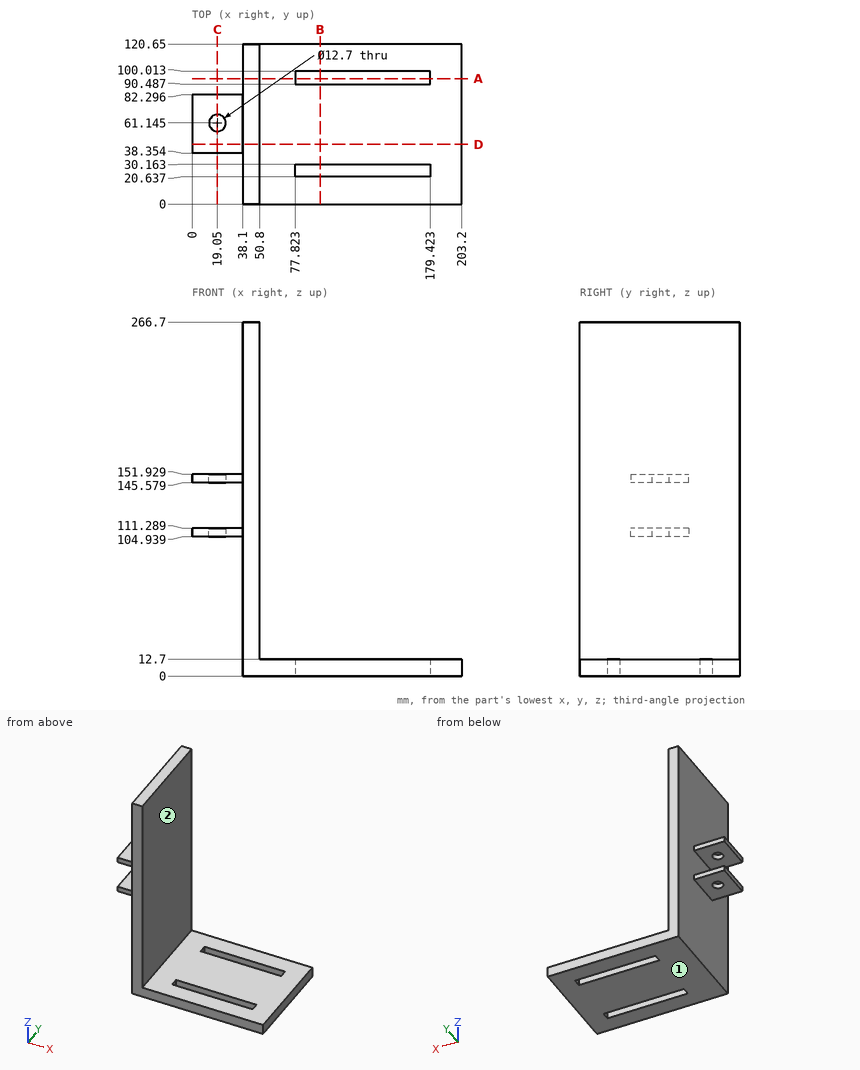
Could you check a few things on this drawing? It's one solid part, dimensions in mm from its lowest x, y, z. A direction names the side the tool comes from. Give positions to 0.01 mm unless a question says otherwise; leave off trailing zeros. Write each loop counter-clockwise with the first axis right and the second up, starting at its lowest first coordinate (ties: lowest second). Pieces come first, ordered by that corner, then holes. Notation, with made-up numbers: M 17.25,73 L 30.25,73 A24 cw 30.25,111 Z; hole C -18,-33 d4. An arc over 180 degrees is marked long. Put each result on its own line as item: value. Start each with the question number.
Item 1: If we section it at A-A, the plane y = 94.5: Write out the boundary of the cut face in (x, z), then the cut area to 3 significant figures.
Item 2: Will these pins go through, and if not, where does the flat tip stop? pin 1 (20.5 mm diameter, centred on x = 19.05, y = 61.15, fed in from +Z); pin 2 (19 mm diameter, centred on x = 26.5, y = 55, fed in from -Z); pin 3 (7 mm diameter, centred on x = 22, z = 108.5, fed in from -Y).
Item 3: If we section it at B-B, the plane x = 96.5: Write out the boundary of the cut face in (y, z), then the cut area to 3 significant figures.
Item 4: On a 3-axis mill with a long thin cutter (end or side, diameter ignored), from which of +Z, -Z, +X, -X, +Y, -Y can I reach the whole of each face in a straight line? I mean the marked faces 1 and 2. Say none if no direction works.
Item 5: I need wall thicknesses on L1, parallel to Y at x = 19.05, z = 149.25 (1 decimal); L2, parallel to X at y = 79, z = 162.5; L3, parallel to Z at x = 143, y = 30.5. Which ranges of each line are inside material? Lowest first, please. Write a range as from..to.
Item 6: If we section it at D-D, the plane y = 45: Write out the boundary of the cut face in (x, z), then the cut area to 3 significant figures.
Item 7: If we section it at C-C, the plane x = 19.05: Write out the boundary of the cut face in (y, z) (1 decimal).
Values:
1. outline: M 38.1,0 L 77.82,0 L 77.82,12.7 L 50.8,12.7 L 50.8,266.7 L 38.1,266.7 Z; M 179.42,0 L 203.2,0 L 203.2,12.7 L 179.42,12.7 Z
1. area: 4,030 mm²
2. pin 1: z = 151.93
2. pin 2: z = 104.94
2. pin 3: y = 38.35
3. outline: M 0,0 L 20.64,0 L 20.64,12.7 L 0,12.7 Z; M 30.16,0 L 90.49,0 L 90.49,12.7 L 30.16,12.7 Z; M 100.01,0 L 120.65,0 L 120.65,12.7 L 100.01,12.7 Z
3. area: 1,290 mm²
4. face 1: -Z, +X, -X, +Y, -Y
4. face 2: +Z, +X, +Y, -Y
5. L1: 38.4..54.8, 67.5..82.3
5. L2: 38.1..50.8
5. L3: 0..12.7
6. outline: M 0,104.94 L 38.1,104.94 L 38.1,0 L 203.2,0 L 203.2,12.7 L 50.8,12.7 L 50.8,266.7 L 38.1,266.7 L 38.1,151.93 L 0,151.93 L 0,145.58 L 38.1,145.58 L 38.1,111.29 L 0,111.29 Z
6. area: 5,810 mm²
7. outline: M 38.4,104.9 L 54.8,104.9 L 54.8,111.3 L 38.4,111.3 Z; M 38.4,145.6 L 54.8,145.6 L 54.8,151.9 L 38.4,151.9 Z; M 67.5,104.9 L 82.3,104.9 L 82.3,111.3 L 67.5,111.3 Z; M 67.5,145.6 L 82.3,145.6 L 82.3,151.9 L 67.5,151.9 Z
